Build history of the part. All positions in model axes, mm. A direction names the side the tool comes from. Round coordinates to 2 decimals unless told otherwise and drop trailing zeros. Loops run counter-clockwise (first coordinate to the right, second up) from the corner with the lowest first, then second, coordinate; pieces in that order, holes last. Notation, with made-up numbers: M -33.75,-27 L 25.25,-27 A25 ccw 25.25,11 Z; hole C 76,4 d3. An arc over 180 degrees is marked long. Write each question's results on one line, items separated by ' | '. Start each with the question number.
```python
from build123d import *

# Parameters (mm, degrees)
SKETCH_R        = 150
PAD_DEPTH       = 5
SKETCH001_R     = 4
POCKET_DEPTH    = 5.001
SKETCH003_R     = 20
SKETCH003_R_2   = 4.5
POCKET001_DEPTH = 5
POCKET002_DEPTH = 5
SKETCH004_R     = 4
POCKET003_DEPTH = 5
SKETCH005_R     = 24
SKETCH005_R_2   = 20.5
PAD001_DEPTH    = 60


with BuildPart() as part:
    # Sketch → Pad (new body)
    with BuildSketch(Plane.XY):
        Circle(SKETCH_R)
    extrude(amount=PAD_DEPTH)

    # Sketch001 (on Face3 of Pad) → Pocket (cut, through all)
    with BuildSketch(Plane.XY.offset(5)):
        with Locations((0, 142.5)):
            Circle(SKETCH001_R)
        with Locations((-142.5, 0)):
            Circle(SKETCH001_R)
        with Locations((0, -142.5)):
            Circle(SKETCH001_R)
        with Locations((142.5, 0)):
            Circle(SKETCH001_R)
    extrude(amount=-POCKET_DEPTH, mode=Mode.SUBTRACT)

    # Sketch003 (on Face3 of Pocket) → Pocket001 (cut)
    with BuildSketch(Plane.XY.offset(5)):
        with Locations((0, -62.5)):
            Circle(SKETCH003_R)
        with Locations((0, 32.5)):
            Circle(SKETCH003_R_2)
        with Locations((-38, -37.5)):
            Circle(SKETCH003_R_2)
        with Locations((38, -37.5)):
            Circle(SKETCH003_R_2)
    extrude(amount=-POCKET001_DEPTH, mode=Mode.SUBTRACT)

    # Sketch003 (on Face3 of Pocket) → Pocket002 (cut)
    with BuildSketch(Plane.XY.offset(5)):
        with Locations((0, -62.5)):
            Circle(SKETCH003_R)
        with Locations((0, 32.5)):
            Circle(SKETCH003_R_2)
        with Locations((-38, -37.5)):
            Circle(SKETCH003_R_2)
        with Locations((38, -37.5)):
            Circle(SKETCH003_R_2)
    extrude(amount=-POCKET002_DEPTH, mode=Mode.SUBTRACT)

    # Sketch004 (on Face3 of Pocket002) → Pocket003 (cut)
    with BuildSketch(Plane.XY.offset(5)):
        with Locations((100.763433, 100.762)):
            Circle(SKETCH004_R)
        with Locations((100.762, -100.763433)):
            Circle(SKETCH004_R)
        with Locations((-54.532, -131.652995)):
            Circle(SKETCH004_R)
        with Locations((-100.763433, 100.762)):
            Circle(SKETCH004_R)
        with Locations((-100.762, -100.763433)):
            Circle(SKETCH004_R)
        with Locations((-131.652995, -54.532)):
            Circle(SKETCH004_R)
        with Locations((-131.652995, 54.532)):
            Circle(SKETCH004_R)
        with Locations((-54.532, 131.652995)):
            Circle(SKETCH004_R)
        with Locations((54.532, 131.652995)):
            Circle(SKETCH004_R)
        with Locations((131.740607, 54.32)):
            Circle(SKETCH004_R)
        with Locations((54.532, -131.652995)):
            Circle(SKETCH004_R)
        with Locations((131.652995, -54.532)):
            Circle(SKETCH004_R)
    extrude(amount=-POCKET003_DEPTH, mode=Mode.SUBTRACT)

    # Sketch005 (on Face3 of Pocket003) → Pad001 (join)
    with BuildSketch(Plane.XY.offset(5)):
        with Locations((0, -62.5)):
            Circle(SKETCH005_R)
        with Locations((0, -62.5)):
            Circle(SKETCH005_R_2, mode=Mode.SUBTRACT)
    extrude(amount=PAD001_DEPTH)


solid = part.part
```
Item 1: Drop flat-ended pins along their axis: pin 1 (13 mm diameter, centred on x = -131.65, y = -54.53, fed in from +Z); pin 2 (2 mm diameter, centred on y = -83.5, z = 43, fed in from -X); pin 3 (12 mm diameter, centred on x = 1.5, z = 23.5, fed in from +Y). Give the stop position or say it passes through.
Item 2: Mould opens along X. For faces 3 (the flat face through (-2, 2, 5)), 4 (the cylindrical face through (-3.1, -38.7, 34.6)), 5 (the cylindrical face through (128.79, 57.02, 2.54)) say: released by +X, released by -X, zero draft, split by the parting line, or undercut.
Item 3: Saw through at B-B, the plane y = -142.5. Give the cut face in (x, z), then the cut area to 3 significant figures.
Item 4: Tool access for faces 1 (the cylindrical face through (135.47, -53.33, 2.54)), 2 (the cylindrical face through (9.459, -80.687, 34.58)): list every direction of +Z, -Z, +X, -X, +Y, -Y with a clear straight run to the whole face (end or side of a thin tool).
Item 5: Drill centre lines: line 1 along Y through (x, z) = (0, 2.55); line 2 along X through (y, z) = (-63.5, 38); line 3 along Z through (x, y) = (117.5, 18). Where is each one in solid material? Low to high. Write a range as [from, to].
Item 6: Saw through at A-A, the plane x = 0. Give the cut face in (y, z).
Item 7: Saw through at D-D, the plane z = 30. Give the cut face in (x, y), then the cut area to 3 significant figures.
Working result:
1) pin 1: stops at z = 5 | pin 2: stops at x = -13.27 | pin 3: stops at y = -38.5
2) face 3: zero draft | face 4: split by the parting line | face 5: undercut
3) outline: M -46.84,0 L -4,0 L -4,5 L -46.84,5 Z; M 4,0 L 46.84,0 L 46.84,5 L 4,5 Z | area: 428 mm²
4) face 1: +Z, -Z | face 2: +Z
5) line 1: y = [-150, -146.5], [-138.5, -82.5], [-42.5, 28], [37, 138.5], [146.5, 150] | line 2: x = [-23.98, -20.48], [20.48, 23.98] | line 3: z = [0, 5]
6) outline: M -150,0 L -146.5,0 L -146.5,5 L -150,5 Z; M -138.5,0 L -82.5,0 L -82.5,5 L -83,5 L -83,65 L -86.5,65 L -86.5,5 L -138.5,5 Z; M -42.5,0 L 28,0 L 28,5 L -38.5,5 L -38.5,65 L -42,65 L -42,5 L -42.5,5 Z; M 37,0 L 138.5,0 L 138.5,5 L 37,5 Z; M 146.5,0 L 150,0 L 150,5 L 146.5,5 Z
7) outline: C 0,-62.5 d48; hole C 0,-62.5 d41 | area: 489 mm²
